from build123d import *


with BuildPart() as f2:
    # F2: sweep along a path in F0
    with BuildLine(Plane.XZ) as f2_path:
        CenterArc((0, 0), 4, 0, 360)
    # F1 (on Right) → F2 (sweep)
    with BuildSketch(Plane.YZ):
        Polygon((0, 7), (0, 4), (24, 4), (24, 7), (23.5, 7.5), (20.75, 7.5), (20.75, 7.15), (19.65, 7.15), (19.65, 7.5), (12, 7.5), (4.35, 7.5), (4.35, 7.15), (3.25, 7.15), (3.25, 7.5), (0.5, 7.5), align=None)
    sweep(path=f2_path.line)


solid = f2.part
Read the model definition and answer for the solid it produces. Units are mm, in the model's axes. A direction names the side the tool comes from. Round coordinates to 2 decimals unless told otherwise and drop trailing zeros.
1) Flat-ended cylindrical pins translate along their axes: pin 1 (4 mm diameter, centred on x = -0.5, y = 3, fed in from -Z); pin 2 (1 mm diameter, centred on x = 5, y = 17, fed in from +Z); pin 3 (7 mm diameter, centred on x = 0, z = 0, fed in from -Y); pin 4 (1.5 mm diameter, centred on x = 3.5, y = 9, fed in from -Z). Find the tip coordinate at first contact, or state that the pin passes through.
2) Straight lines are drawn through the part: L1, parallel to Z at x = 0, y = 5; L2, parallel to Y at x = -4.25, z = -6; L3, parallel to Z at x = -3.5, y = 6.25. For each, find the intervals that lie inside material, in ascending order.
3) For faces 3 (the face through (-0.867, 12.168, -3.905)), 4 (the face through (-0.93, 3.79, 7.09)), determine the directions among +Z, -Z, +X, -X, +Y, -Y from which every point of the face is accessible in a straight line to the end or side of a thin tool.
4) The mould has two halves that part along Y. Classify faces 1 (the face through (-0.93, 20.19, 7.09)), 2 (the face through (-1.63, 11.89, -7.32)): released by +Y, released by -Y, zero draft, split by the parting line, or undercut.
Resolved:
1. pin 1: stops at z = -7.5
1. pin 2: stops at z = 6
1. pin 3: passes through
1. pin 4: stops at z = -6.98
2. L1: z = -7.5 to -4, 4 to 7.5
2. L2: y = 0.35 to 3.25, 4.35 to 19.65, 20.75 to 23.65
2. L3: z = -6.63 to -1.94, 1.94 to 6.63
3. face 3: +Y, -Y
3. face 4: none
4. face 1: undercut
4. face 2: zero draft
